Here's how the part is built. I have some questions about the finished solid (model axes, mm). A direction names the side the tool comes from. Coordinates: 2 decimals unless noted, no trailing zeros. Order: outer loops, then holes, each group sorted by start corner. A loop starts at its lowest first (then second) coordinate and runs counter-clockwise, first axis right, second up. Notation, with made-up numbers: (2, 10.25) - (40, 10.25) arc R9 ccw to (40, 23.25) - close; hole circle Ø11 at (-9, -6.5). An arc over 180 degrees is marked (long way). Use one line per item in the form item = value. Start each with the question number.
from build123d import *

# Parameters (mm, degrees)
EXTRUDE_8_DEPTH = 20
SKETCH_1_R      = 14.8
EXTRUDE_1_DEPTH = 60
SKETCH_2_R      = 3
EXTRUDE_2_DEPTH = 5


with BuildPart() as part:
    # 草图3 → 凸台-拉伸8 (new body)
    with BuildSketch(Plane(origin=(0, 20, 0), x_dir=(1, 0, 0), z_dir=(0, 1, 0))):
        with BuildLine():
            Line((0, 48), (90, 48))
            ThreePointArc((90, 48), (102.727922061, 42.727922061), (108, 30))
            Line((108, 30), (108, 0))
            ThreePointArc((108, 0), (102.727922061, -12.727922061), (90, -18))
            Line((90, -18), (0, -18))
            ThreePointArc((0, -18), (-12.727922061, -12.727922061), (-18, 0))
            Line((-18, 0), (-18, 30))
            ThreePointArc((-18, 30), (-12.727922061, 42.727922061), (0, 48))
        make_face()
    extrude(amount=EXTRUDE_8_DEPTH)

    # 草图1 → 凸台-拉伸1 (add)
    with BuildSketch(Plane(origin=(0, 0, 0), x_dir=(1, 0, 0), z_dir=(0, 1, 0))):
        with Locations(Location((0, 30, 0), (0, 0, 270))):
            Circle(SKETCH_1_R)
        with Locations(Location((30, 30, 0), (0, 0, 270))):
            Circle(SKETCH_1_R)
        with Locations(Location((60, 30, 0), (0, 0, 270))):
            Circle(SKETCH_1_R)
        with Locations(Location((90, 30, 0), (0, 0, 270))):
            Circle(SKETCH_1_R)
        with Locations(Location((90, 0, 0), (0, 0, 270))):
            Circle(SKETCH_1_R)
        with Locations(Location((60, 0, 0), (0, 0, 270))):
            Circle(SKETCH_1_R)
        with Locations(Location((30, 0, 0), (0, 0, 270))):
            Circle(SKETCH_1_R)
        with Locations(Location((0, 0, 0), (0, 0, 270))):
            Circle(SKETCH_1_R)
    extrude(amount=EXTRUDE_1_DEPTH)

    # 草图2 → 凸台-拉伸2 (add)
    with BuildSketch(Plane(origin=(0, 60, 0), x_dir=(1, 0, 0), z_dir=(0, 1, 0))):
        with Locations(Location((0, 30, 0), (0, 0, 270))):
            Circle(SKETCH_2_R)
        with Locations(Location((30, 30, 0), (0, 0, 270))):
            Circle(SKETCH_2_R)
        with Locations(Location((60, 30, 0), (0, 0, 270))):
            Circle(SKETCH_2_R)
        with Locations(Location((90, 30, 0), (0, 0, 270))):
            Circle(SKETCH_2_R)
        with Locations(Location((30, 0, 0), (0, 0, 270))):
            Circle(SKETCH_2_R)
        with Locations(Location((60, 0, 0), (0, 0, 270))):
            Circle(SKETCH_2_R)
        with Locations(Location((90, 0, 0), (0, 0, 270))):
            Circle(SKETCH_2_R)
        with Locations(Location((0, 0, 0), (0, 0, 270))):
            Circle(SKETCH_2_R)
    extrude(amount=EXTRUDE_2_DEPTH)


solid = part.part
1) Suppose I cut it at A-A, the plane y = 7. List the corners of the cut face in (x, z) for me.
2) Suppose I cut it at D-D, the plane x = -6. List the corners of the cut face in (y, z) for me, then the cut area to 3 significant figures.
3) If we mould it in two halves opening along Z, with no side actions, what happens to faces 1 (the flat face through (46, 30, 18)), 2 (the cylindrical face through (64.446, 9.86, 14.117)), 3 (the flat face through (30, 0, -30)), 4 (the cylindrical face through (62.53, 62.46, 1.61))? For each: pulls with the +Z half, pulls with the -Z half, needs draft (parallel to the pull), parting line crosses it, or undercut.
4) Suppose I cut it at C-C, the plane y = 34. List the corners of the cut face in (x, z) for me.
5) Which directions (+Z, -Z, +X, -X, +Y, -Y) give clear straight access to the entire face, cutting with the end or side of a thin tool? Please do faces 5 (the cylindrical face through (-14.448, 9.86, -3.208)), 6 (the cylindrical face through (44.674, 49.86, -1.927)), 7 (the cylindrical face through (102.587, 29.86, -42.867)).
6) I need wall thicknesses on probe 1 along X at (y, z) = (4, -43); probe 2 along X at (y, z) = (48, 3); probe 3 along Y at (x, z) = (55, -37). Which ranges of each line are inside material? Lowest first, please. Write a range as [from, to].
7) For pin 1 (20 mm diameter, centred on x = 36, z = -13, fed in from +Y); pin 2 (2 mm diameter, centred on x = 16, y = 18, fed in from +Z); pin 3 (6 mm diameter, centred on y = 52, z = -38.5, fed in from +X), each with a flat end and sliding along its axis, tell me the tip position at first contact or that it passes through.
8) Suppose I cut it at B-B, the plane x = 60. List the corners of the cut face in (y, z) for me, then the cut area to 3 significant figures.
From the geometry:
q1.outline = circle Ø29.6 at (0, -30); circle Ø29.6 at (0, 0); circle Ø29.6 at (30, -30); circle Ø29.6 at (30, 0); circle Ø29.6 at (60, -30); circle Ø29.6 at (60, 0); circle Ø29.6 at (90, -30); circle Ø29.6 at (90, 0)
q2.outline = (0, -43.53) - (20, -43.53) - (20, -46.97) - (40, -46.97) - (40, -43.53) - (60, -43.53) - (60, -16.47) - (40, -16.47) - (40, -13.53) - (60, -13.53) - (60, 13.53) - (40, 13.53) - (40, 16.97) - (20, 16.97) - (20, 13.53) - (0, 13.53) - (0, -13.53) - (20, -13.53) - (20, -16.47) - (0, -16.47) - close
q2.area = 3,440 mm2
q3.face_1 = pulls with the +Z half
q3.face_2 = undercut
q3.face_3 = needs draft
q3.face_4 = undercut
q4.outline = (-18, -30) arc R18 ccw to (0, -48) - (90, -48) arc R18 ccw to (108, -30) - (108, 0) arc R18 ccw to (90, 18) - (0, 18) arc R18 ccw to (-18, 0) - close
q5.face_5 = -Y
q5.face_6 = +Y
q5.face_7 = -Z, +X, +Y, -Y
q6.probe_1 = [-7.07, 7.07], [22.93, 37.07], [52.93, 67.07], [82.93, 97.07]
q6.probe_2 = [-14.49, 14.49], [15.51, 44.49], [45.51, 74.49], [75.51, 104.49]
q6.probe_3 = [0, 60]
q7.pin_1 = 60
q7.pin_2 = 7.07
q7.pin_3 = 103.74
q8.outline = (0, -44.8) - (20, -44.8) - (20, -48) - (40, -48) - (40, -44.8) - (60, -44.8) - (60, -33) - (65, -33) - (65, -27) - (60, -27) - (60, -15.2) - (40, -15.2) - (40, -14.8) - (60, -14.8) - (60, -3) - (65, -3) - (65, 3) - (60, 3) - (60, 14.8) - (40, 14.8) - (40, 18) - (20, 18) - (20, 14.8) - (0, 14.8) - (0, -14.8) - (20, -14.8) - (20, -15.2) - (0, -15.2) - close
q8.area = 3,750 mm2
